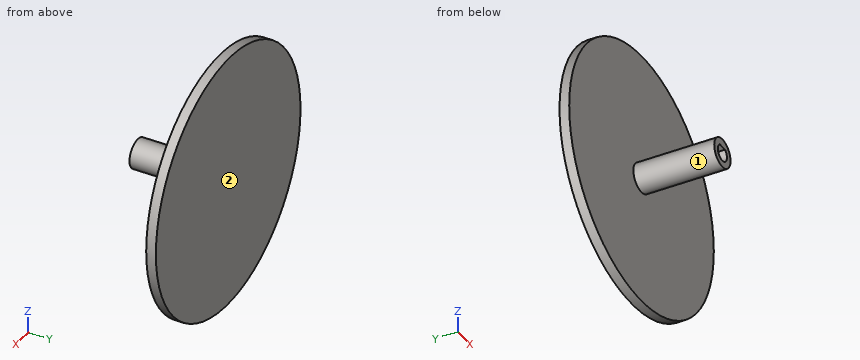
Autodesk Inventor part; units mm, degrees
ref_plane "YZ Plane" through (0, 0, 0) normal (1, 0, 0) x (0, 1, 0)
ref_plane "XZ Plane" through (0, 0, 0) normal (0, 1, 0) x (-1, 0, 0)
ref_plane "XY Plane" through (0, 0, 0) normal (0, 0, 1) x (1, 0, 0)
sketch "Sketch1" plane through (0, 0, 0) normal (0, 1, 0) x (-1, 0, 0)
  circle A0 centre (0, 0) radius 4.5
  arc A1 (-1.5, 2) -> (1.5, 2) centre (0, 0) ccw
  line L0 (1.5, 2) -> (-1.5, 2)
  arc A2 (1.5, 2) -> (-1.5, 2) centre (0, 0) ccw construction
  dimension "d0" = 5
  dimension "d1" = 9
  dimension "d4" = 3
extrude "Extrusion1" add sketch "Sketch1" against normal blind 25
sketch "Sketch2" plane through (0, 0, 0) normal (0, -1, 0) x (-1, 0, 0)
  circle A0 centre (0, 0) radius 40
  dimension "d5" = 80
extrude "Extrusion2" add sketch "Sketch2" against normal blind 3
extrude "Extrusion3" add sketch "Sketch1" against normal blind 5 contours L0 A1
properties part number "Soporte_mesa"
For this review, take the finished solid that the model builds, in its own axes (mm). Face numbers are marked on the shaded views. A direction names the side the tool comes from. Round coordinates to 2 decimals unless told otherwise and drop trailing zeros. Write each loop counter-clockwise with the first axis right and the second up, starting at its lowest first coordinate (ties: lowest second). Pieces come first, ordered by that corner, then holes.
1) Take a section at D-D on z = -24. Give the boundary of the cut face in (x, y).
Answer below:
outline: (-32, 0) - (32, 0) - (32, 3) - (-32, 3) - close
2) Take a section at C-C on y = -15.75. Give the boundary of the cut face in (x, z).
Answer below:
outline: circle Ø9 at (0, 0); hole (-1.5, 2) arc R2.5 ccw (long way) to (1.5, 2) - close
3) Machinability: for the marked faces 1 and 2, which of the approach directions +Z, -Z, +X, -X, +Y, -Y give a long, thin tool a straight path to every point of the face, cutting with its end or side? Answer none if there is none.
Answer below:
face 1: -Y
face 2: +Z, -Z, +X, -X, +Y
4) Take a section at A-A on x = 0. Give the boundary of the cut face in (y, z), then the cut area to 3 significant figures.
Answer below:
outline: (-25, -4.5) - (0, -4.5) - (0, -40) - (3, -40) - (3, 40) - (0, 40) - (0, 4.5) - (-25, 4.5) - (-25, 2) - (-5, 2) - (-5, -2.5) - (-25, -2.5) - close
area: 375 mm2
5) For line 1 along Z through (x, y) = (0, -15.5); line 2 along Y through (x, z) = (-8.5, 21.5); line 3 along X through (y, z) = (-22.5, -0.5), list the stretches that pass through material, from the lowest coordinate up.
Answer below:
line 1: z = -4.5 to -2.5, 2 to 4.5
line 2: y = 0 to 3
line 3: x = -4.47 to -2.45, 2.45 to 4.47
6) Insertion check: pin 1 Ø3 at (x, z) = (0, 0) entering from -Y; pin 2 Ø10 at (x, z) = (18.5, 31.5) entering from -Y; pin 3 Ø1.5 at (x, y) = (0, -15.5) entering from -Z; pin 4 Ø5 at (y, z) = (-3.5, 11.5) entering from +X. Each pin has a flat end and moves straight along its axis. Give the tip position at first contact, or say it passes through.
Answer below:
pin 1: stops at y = -5
pin 2: stops at y = 0
pin 3: stops at z = -4.5
pin 4: passes through
7) Take a section at B-B on z = 0. Give the boundary of the cut face in (x, y).
Answer below:
outline: (-40, 0) - (-4.5, 0) - (-4.5, -25) - (-2.5, -25) - (-2.5, -5) - (2.5, -5) - (2.5, -25) - (4.5, -25) - (4.5, 0) - (40, 0) - (40, 3) - (-40, 3) - close
